The model under review builds one solid part; all positions refer to its coordinate system, in mm. A direction names the side the tool comes from. Coordinates: 2 decimals unless noted, no trailing zeros. Order: outer loops, then holes, each group sorted by start corner. A loop starts at its lowest first (then second) coordinate and runs counter-clockwise, first axis right, second up.
```python
from build123d import *

# Parameters (mm, degrees)
F2_SIZE = 0.2


with BuildPart() as f1:
    # F0 (on Front) → F1 (revolve)
    with BuildSketch(Plane.XZ):
        Polygon((8, 43), (4.1, 43), (4.1, 32.5), (2.1, 31.298279), (2.1, 17.040775), (3, 16.5), (3, 0), (11.1, 0), (11.1, 1.5), (4.1, 1.5), (4.1, 3), (11.1, 3), (11.1, 4), (4.1, 4), (4.1, 5.5), (11.1, 5.5), (11.1, 6.5), (4.1, 6.5), (4.1, 8), (11.1, 8), (11.1, 9), (4.1, 9), (4.1, 10.5), (11.1, 10.5), (11.1, 11.5), (4.1, 11.5), (4.1, 13), (11.1, 13), (11.1, 14), (4.1, 14), (4.1, 15.5), (11.1, 15.5), (11.1, 16.5), (4.1, 16.5), (4.1, 18), (11.1, 18), (11.1, 19), (4.1, 19), (4.1, 20.5), (11.1, 20.5), (11.1, 21.5), (4.1, 21.5), (4.1, 23), (11.1, 23), (11.1, 24), (4.1, 24), (4.1, 25.5), (11.1, 25.5), (11.1, 26.5), (4.1, 26.5), (4.1, 28), (8, 28), (8, 29), (4.1, 29), (4.1, 30.5), (8, 30.5), (8, 33), (6, 33), (6, 39), (8, 39), align=None)
    revolve(axis=Axis((0, 0, 21.5), (0, 0, 1)))

    # F2
    f2_edges = [f1.edges().sort_by_distance(p)[0] for p in [
        (-8, 0, 30.5),
        (-8, 0, 33),
        (-8, 0, 39),
        (-8, 0, 43),
    ]]
    chamfer(f2_edges, length=F2_SIZE)


solid = f1.part
```
(1) Draft analysis for pull direction Y (two halves, no side actions). For faces 4 (the face through (-5, 0, 10.5)), 5 (the face through (-0.534, 4.065, 37.676)), 6 (the face through (5.97, 9.36, 8.51)), state which applies: released by +Y, released by -Y, zero draft, split by the parting line, or undercut.
A:
face 4: zero draft
face 5: undercut
face 6: split by the parting line
(2) We need section A-A, the plane z = 34. Write out the cut boundary in (x, y), and give its area (3 significant figures).
A:
outline: circle Ø12 at (0, 0); hole circle Ø8.2 at (0, 0)
area: 60.3 mm2
(3) Wall thickness on probe 1 along Y at (x, z) = (0, 40.5); probe 2 along Y at (x, z) = (0, 27); probe 3 along X at (y, z) = (-1.5, 10): over which ranges is each line inside the solid? List them lowest first.
A:
probe 1: y = -8 to -4.1, 4.1 to 8
probe 2: y = -4.1 to -2.1, 2.1 to 4.1
probe 3: x = -3.82 to -2.6, 2.6 to 3.82
(4) For pin 1 Ø6 at (x, z) = (-8.5, 32) entering from +Y; pin 2 Ø4 at (y, z) = (9, 26.5) entering from -X; pin 3 Ø1 at (y, z) = (-7, 11.5) entering from -X, all flat-tipped, find the tip position at first contact; note any pin that passes through.
A:
pin 1: stops at y = 5.81
pin 2: stops at x = -8.61
pin 3: stops at x = -9
(5) Machinability: for faces 1 (the face through (-1.73, -7.81, 28.51)), 2 (the face through (-3, 0, 8)), 3 (the face through (5, 0, 21.5)), which of the approach directions +Z, -Z, +X, -X, +Y, -Y give a long, thin tool a straight path to every point of the face, cutting with its end or side? Answer none if there is none.
A:
face 1: +Z
face 2: -Z
face 3: none
(6) We need section B-B, the plane y = 8.75. Count the separate pieces of the cut face and the enclosed holes in it, and give its area (3 significant figures).
A:
separate pieces: 11
enclosed holes: 0
area: 157 mm2
